Geometry check sheet. Reference: the model listing, model coordinates, mm. Face numbers are marked on the shaded views. Round coordinates to 2 decimals unless told otherwise and drop trailing zeros. Loops run counter-clockwise (first coordinate to the right, second up) from the corner with the lowest first, then second, coordinate; pieces in that order, holes last. Notation, with made-up numbers: (18.25, 27.5) -> (56.25, 27.5) arc R25 ccw to (56.25, 59.5) -> close; hole circle Ø8 at (-22, -38.75). An arc over 180 degrees is marked (long way). Use a Markdown table: item, result. Add a question column.
Q1. Sectioned sample at B-B, the plane y = 112.5. Enter the section's corners in (x, z), then the cut area to 3 significant figures.
Q2. Sectioned sample at A-A, the plane x = 32. Enter the section's corners in (y, z).
Q3. Material ranges on L1, parallel to X at y = -0.5, z = 103; L2, parallel to Y at x = 89, z = -312; L3, parallel to Z at x = 81, y = 130, recorded low to high.
Q4. Sectioned sample at C-C, the plane z = -246. Enter the section's corners in (x, y), then the cut area to 3 significant figures.
Q5. Release check for a two-part mould opening along X. For the marked faces 1, 2 and 3 record: released by +X, released by -X, zero draft, split by the parting line, or undercut.
Q6. Sectioned sample at D-D, the plane z = -28. Enter the section's corners in (x, y), then the cut area to 3 significant figures.
Q7. Gauge pin test, flat ends, axial feed: P1, Ø4, axis at y = 71.5, z = -217, coming from the -X side; P2, Ø1.5, axis at y = 62, z = -1.5, coming from the -X side; P3, Ø10, axis at y = -15, z = -194, coming from the -X side; P4, Ø18.5, axis at x = 85, y = 31.5, coming from the -Z side. Record the tip position at first contact, or that the pin passes through.
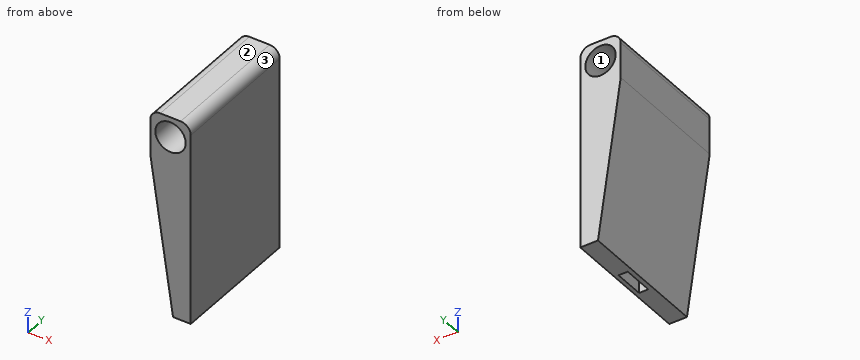
```python
from build123d import *

# Parameters (mm, degrees)
SKETCH2_W           = 508
SKETCH2_H           = 330.2
BOSS_EXTRUDE1_DEPTH = 101.6
SKETCH3_R           = 38.1
CUT_EXTRUDE1_DEPTH  = 331.2
FILLET1_R           = 25.4
CUT_EXTRUDE2_DEPTH  = 331.2
SKETCH5_W           = 23.104275201
SKETCH5_H           = 76.2
CUT_EXTRUDE3_DEPTH  = 50.8


with BuildPart() as part:
    # Sketch2 → Boss-Extrude1 (new body)
    with BuildSketch(Plane(origin=(0, 0, 0), x_dir=(0, 0, -1), z_dir=(1, 0, 0))):
        with Locations((98.635814889, 33.244869215)):
            Rectangle(SKETCH2_W, SKETCH2_H)
    extrude(amount=BOSS_EXTRUDE1_DEPTH)

    # Sketch3 → Cut-Extrude1 (cut, through all)
    with BuildSketch(Plane.XZ.offset(131.855130785)):
        with Locations((50.8, 104.564185111)):
            Circle(SKETCH3_R)
    extrude(amount=-CUT_EXTRUDE1_DEPTH, mode=Mode.SUBTRACT)

    # Fillet1
    fillet1_edges = [part.edges().sort_by_distance(p)[0] for p in [
        (101.6, 33.244869215, 155.364185111),
        (0, 33.244869215, 155.364185111),
    ]]
    fillet(fillet1_edges, radius=FILLET1_R)

    # Sketch4 → Cut-Extrude2 (cut, through all)
    with BuildSketch(Plane.XZ.offset(131.855130785)):
        Polygon((0, 40.959246462), (57.15, -352.635814889), (0, -352.635814889), align=None)
    extrude(amount=-CUT_EXTRUDE2_DEPTH, mode=Mode.SUBTRACT)

    # Sketch5 → Cut-Extrude3 (cut)
    with BuildSketch(Plane(origin=(0, 0, -352.635814889), x_dir=(-1, 0, 0), z_dir=(0, 0, -1))):
        with Locations((-79.8878624, 33.244869215)):
            Rectangle(SKETCH5_W, SKETCH5_H)
    extrude(amount=-CUT_EXTRUDE3_DEPTH, mode=Mode.SUBTRACT)


solid = part.part
```
Values:
| question | item | result |
|---|---|---|
| 1 | outline | (0, 40.96) -> (57.15, -352.64) -> (101.6, -352.64) -> (101.6, 129.96) arc R25.4 ccw to (76.2, 155.36) -> (25.4, 155.36) arc R25.4 ccw to (0, 129.96) -> close; hole circle Ø76.2 at (50.8, 104.56) |
| 1 | area | 35,500 mm^2 |
| 2 | outline | (-131.86, -179.43) -> (198.34, -179.43) -> (198.34, 71.43) -> (-131.86, 71.43) -> close; (-131.86, 137.7) -> (198.34, 137.7) -> (198.34, 155.36) -> (-131.86, 155.36) -> close |
| 3 | L1 | 0 to 12.73, 88.87 to 101.6 |
| 3 | L2 | -131.86 to -4.86, 71.34 to 198.34 |
| 3 | L3 | -352.64 to 81.34, 127.79 to 154.91 |
| 4 | outline | (41.67, -131.86) -> (101.6, -131.86) -> (101.6, 198.34) -> (41.67, 198.34) -> close |
| 4 | area | 19,800 mm^2 |
| 5 | face 1 | undercut |
| 5 | face 2 | zero draft |
| 5 | face 3 | released by +X |
| 6 | outline | (10.01, -131.86) -> (101.6, -131.86) -> (101.6, 198.34) -> (10.01, 198.34) -> close |
| 6 | area | 30,200 mm^2 |
| 7 | P1 | x = 37.17 |
| 7 | P2 | x = 6.06 |
| 7 | P3 | x = 33.39 |
| 7 | P4 | z = -352.64 |
